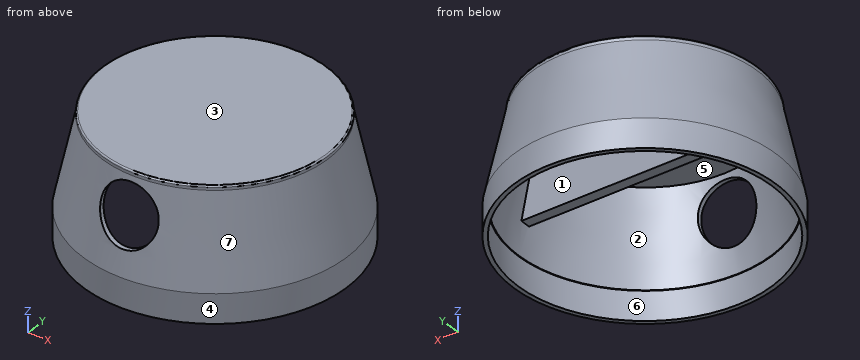
```python
from build123d import *

# Parameters (mm, degrees)
SKETCH2_R                       = 77.5
SKETCH1_R                       = 90.55
SKETCH4_R                       = 74.5
SKETCH3_R                       = 87.05
SKETCH5_R                       = 77.5
BOSS_EXTRUDE1_DEPTH             = 3
SKETCH7_R                       = 20
CUT_EXTRUDE1_DEPTH              = 159
BOSS_EXTRUDE4_REACH             = 144.715
SKETCH9_W                       = 30.851346151
SKETCH9_H                       = 7.25914027
BOSS_EXTRUDE4_DIRECTION_2_REACH = 144.715
FILLET2_R                       = 1
SKETCH1_7_R                     = 90.55
SKETCH1_7_R_2                   = 87.55
BOSS_EXTRUDE6_DEPTH             = 20


with BuildPart() as part:
    # Sketch2 → Loft2 section 0
    with BuildSketch(Plane.XY.offset(60)):
        Circle(SKETCH2_R)
    # Sketch1 → Loft2 section 1
    with BuildSketch(Plane.XY):
        Circle(SKETCH1_R)
    loft()

    # Sketch4 → Cut-Loft1 section 0
    with BuildSketch(Plane.XY.offset(60)):
        Circle(SKETCH4_R)
    # Sketch3 → Cut-Loft1 section 1
    with BuildSketch(Plane(origin=(0, 0, 0), x_dir=(-1, 0, 0), z_dir=(0, 0, -1))):
        Circle(SKETCH3_R)
    loft(mode=Mode.SUBTRACT)

    # Sketch5 → Boss-Extrude1 (add)
    with BuildSketch(Plane.XY.offset(60)):
        Circle(SKETCH5_R)
    extrude(amount=BOSS_EXTRUDE1_DEPTH)

    # Sketch7 → Cut-Extrude1 (cut)
    with BuildSketch(Plane(origin=(0, 0, 0), x_dir=(1, 0, 0), z_dir=(0, 1, 0))):
        with Locations(Location((0, -36.396883827, 0), (0, 0, 134.764309211))):
            Circle(SKETCH7_R)
    extrude(amount=-CUT_EXTRUDE1_DEPTH, mode=Mode.SUBTRACT)

    # Boss-Extrude4: up to this cone (the profile starts inside it)
    boss_extrude4_end = Plane(origin=(0, 0, 35.178058), z_dir=(0, 0, -1)) * Cone(32.648891502, 126.734954235, 449.813845737, mode=Mode.PRIVATE)
    # Sketch9 → Boss-Extrude4 (add, up to the surface)
    with BuildSketch(Plane(origin=(0, 0, 0), x_dir=(0, 0, -1), z_dir=(1, 0, 0)), mode=Mode.PRIVATE) as boss_extrude4_sk1:
        with Locations((-35.178058342, 0)):
            Rectangle(SKETCH9_W, SKETCH9_H)
    boss_extrude4_tool1 = extrude(boss_extrude4_sk1.sketch, amount=BOSS_EXTRUDE4_REACH, mode=Mode.PRIVATE) & boss_extrude4_end
    add(boss_extrude4_tool1.solids().sort_by_distance((0, 0, 35.178058))[0])

    # Boss-Extrude4 direction 2: up to this cone (the profile starts inside it)
    boss_extrude4_direction_2_end = Plane(origin=(0, 0, 35.178058), z_dir=(0, 0, -1)) * Cone(32.648891502, 126.734954235, 449.813845737, mode=Mode.PRIVATE)
    # Sketch9 → Boss-Extrude4 direction 2 (add, up to the surface)
    with BuildSketch(Plane(origin=(0, 0, 0), x_dir=(0, 0, -1), z_dir=(1, 0, 0)), mode=Mode.PRIVATE) as boss_extrude4_direction_2_sk1:
        with Locations((-35.178058342, 0)):
            Rectangle(SKETCH9_W, SKETCH9_H)
    boss_extrude4_direction_2_tool1 = extrude(boss_extrude4_direction_2_sk1.sketch, amount=-BOSS_EXTRUDE4_DIRECTION_2_REACH, mode=Mode.PRIVATE) & boss_extrude4_direction_2_end
    add(boss_extrude4_direction_2_tool1.solids().sort_by_distance((0, 0, 35.178058))[0])

    # Fillet2
    fillet2_edges = [part.edges().sort_by_distance(p)[0] for p in [
        (-77.5, 0, 63),
    ]]
    fillet(fillet2_edges, radius=FILLET2_R)

    # Sketch1_7 → Boss-Extrude6 (add)
    with BuildSketch(Plane.XY):
        Circle(SKETCH1_7_R)
        Circle(SKETCH1_7_R_2, mode=Mode.SUBTRACT)
    extrude(amount=-BOSS_EXTRUDE6_DEPTH)


solid = part.part
```
Geometry: final body of the model. Coordinates: model frame, mm. Face numbers are marked on the shaded views. A direction names the side the tool comes from. Coordinates: 2 decimals unless noted, no trailing zeros. Order: outer loops, then holes, each group sorted by start corner. A loop starts at its lowest first (then second) coordinate and runs counter-clockwise, first axis right, second up. Notation, with made-up numbers: (82, 55.25) - (133, 55.25) arc R21 ccw to (133, 93.25) - close; hole circle Ø6 at (-23.5, -10). An arc over 180 degrees is marked (long way). Return JSON: item names as keys, results as strings. Group by question number.
1. Pull-direction query (X, two-part tool) for the marked faces 1, 2, 3 and 4; classes: pulls with the +X half, pulls with the -X half, needs draft (parallel to the pull), parting line crosses it, or undercut.
2. Cut plane C-C (z = -12.5). Output: boundary loops of the cut face in (x, y), plus the area to 3 significant figures.
3. Cut plane B-B (z = 38). Output: boundary loops of the cut face in (x, y) (3 decimals).
4. Cut plane A-A (x = 0). Output: boundary loops of the cut face in (y, z).
5. Set-up query: the marked faces 5, 6 and 7. Return all of +Z, -Z, +X, -X, +Y, -Y with unobstructed straight access to the full face (end or side cutting, diameter ignored); none if empty.
6. Pin query (flat end, axial travel): pin 1 (4 mm diameter, centred on x = 65, z = 11.5, fed in from -Y); pin 2 (1 mm diameter, centred on x = -32.5, z = 43, fed in from +Y); pin 3 (1 mm diameter, centred on y = -25.5, z = 45.5, fed in from -X). Return the tip coordinate at first contact, or that it passes through.
Resolved:
{
 "1": {"face 1": "undercut", "face 2": "undercut", "face 3": "needs draft", "face 4": "parting line crosses it"},
 "2": {"outline": "circle Ø181.1 at (0, 0); hole circle Ø175.1 at (0, 0)", "area": "1,680 mm²"},
 "3": {"outline": "(-79.018, -3.63) - (79.018, -3.63) arc R79.102 cw to (19.936, -76.548) - (19.936, -79.834) arc R82.285 ccw (long way) to (-19.936, -79.834) - (-19.936, -76.548) arc R79.102 cw to start; hole (-79.018, 3.63) - (79.018, 3.63) arc R79.102 ccw to start"},
 "4": {"outline": "(-90.55, -20) - (-87.55, -20) - (-87.55, 0) - (-87.05, 0) - (-83.62, 16.4) - (-86.98, 16.4) - (-90.55, 0) - close; (-78.28, 56.4) - (-75.25, 56.4) - (-74.5, 60) - (74.5, 60) - (87.05, 0) - (87.55, 0) - (87.55, -20) - (90.55, -20) - (90.55, 0) - (77.5, 60) - (77.5, 62) arc R1 ccw to (76.5, 63) - (-76.5, 63) arc R1 ccw to (-77.5, 62) - (-77.5, 60) - close; (-3.63, 19.75) - (3.63, 19.75) - (3.63, 50.6) - (-3.63, 50.6) - close"},
 "5": {"face 5": "none", "face 6": "-Z", "face 7": "+Z"},
 "6": {"pin 1": "stops at y = -61.6", "pin 2": "stops at y = 74.66", "pin 3": "stops at x = -76.72"}
}
